```python
from build123d import *

# Parameters (mm, degrees)
SKETCH1_W = 9
SKETCH1_H = 6.9
SKETCH2_W = 6
SKETCH2_H = 3


with BuildPart() as part:
    # Sketch1 → Revolve1 (revolve)
    with BuildSketch(Plane.XY, mode=Mode.PRIVATE) as revolve1_sk:
        with Locations((-1, 7.55)):
            Rectangle(SKETCH1_W, SKETCH1_H)
    revolve(revolve1_sk.sketch.rotate(Axis((0, 0, 0), (1, 0, 0)), 90), axis=Axis((0, 0, 0), (1, 0, 0)))

    # Sketch2 → Cut-Revolve1 (revolve, cut)
    with BuildSketch(Plane.XY, mode=Mode.PRIVATE) as cut_revolve1_sk:
        with Locations((-1, 9.5)):
            Rectangle(SKETCH2_W, SKETCH2_H)
    revolve(cut_revolve1_sk.sketch.rotate(Axis((0, 0, 0), (1, 0, 0)), 90), axis=Axis((0, 0, 0), (1, 0, 0)), mode=Mode.SUBTRACT)


solid = part.part
```
Geometry: final body of the model. Coordinates: model frame, mm. A direction names the side the tool comes from. Coordinates: 2 decimals unless noted, no trailing zeros. Order: outer loops, then holes, each group sorted by start corner. A loop starts at its lowest first (then second) coordinate and runs counter-clockwise, first axis right, second up.
Item 1: Draft query along X for faces 3 (the face through (-4, 8, 2)), 4 (the face through (3.5, 5, 0)), 5 (the face through (-5.5, 5, 0)). Return one class per face: released by +X, released by -X, zero draft, split by the parting line, or undercut.
Answer:
face 3: undercut
face 4: released by +X
face 5: released by -X
Item 2: Section query D-D (y = 6.5). Output: boundary loops of the cut face in (x, z), then the cut area to 3 significant figures.
Answer:
outline: (-5.5, -8.87) - (-4, -8.87) - (-4, -4.66) - (2, -4.66) - (2, -8.87) - (3.5, -8.87) - (3.5, 8.87) - (2, 8.87) - (2, 4.66) - (-4, 4.66) - (-4, 8.87) - (-5.5, 8.87) - close
area: 109 mm2
Item 3: Section query C-C (x = 3). Output: boundary loops of the cut face in (y, z).
Answer:
outline: circle Ø22 at (0, 0); hole circle Ø8.2 at (0, 0)
Item 4: Material intervals for line 1 along Y through (x, z) = (-2.75, 0); line 2 along X through (y, z) = (10, 1.25); line 3 along Z through (x, y) = (0, 0.5), sorted ascending.
Answer:
line 1: y = -8 to -4.1, 4.1 to 8
line 2: x = -5.5 to -4, 2 to 3.5
line 3: z = -7.98 to -4.07, 4.07 to 7.98
Item 5: Access query for faces 1 (the face through (2, 8, 2)), 2 (the face through (-0.937, -4.065, -0.534)). Directions: +Z, -Z, +X, -X, +Y, -Y. A direction counts if a zero-diameter tool reaches every point of the face in a straight line with its end or side. Return the directions, or none.
Answer:
face 1: none
face 2: +X, -X
Item 6: Section query A-A (y = 0). Output: boundary loops of the cut face in (x, z).
Answer:
outline: (-5.5, -11) - (-4, -11) - (-4, -8) - (2, -8) - (2, -11) - (3.5, -11) - (3.5, -4.1) - (-5.5, -4.1) - close; (-5.5, 4.1) - (3.5, 4.1) - (3.5, 11) - (2, 11) - (2, 8) - (-4, 8) - (-4, 11) - (-5.5, 11) - close
Item 7: Contact query for flat-ended pins moving along their axis: P1, Ø1.5, axis at x = -1, z = 7, coming from the +Y side; P2, Ø2, axis at x = 1.5, z = 4.5, coming from the +Y side; P3, Ø4, axis at x = -1, z = -4.5, coming from the +Y side. Output: stop coordinate, or through.
Answer:
P1: stops at y = 4.99
P2: stops at y = 10.38
P3: stops at y = 7.6
